Here's how the part is built. I have some questions about the finished solid (model axes, mm). A direction names the side the tool comes from. Give positions to 0.01 mm unless a question says otherwise; leave off trailing zeros. Loops run counter-clockwise (first coordinate to the right, second up) from the corner with the lowest first, then second, coordinate; pieces in that order, holes last. Notation, with made-up numbers: (37, -24.5) - (46, -24.5) arc R20 cw to (46, 7.5) - close; hole circle Ø8 at (-23, 21.5). An arc over 180 degrees is marked (long way). Use one line per item in the form item = value.
from build123d import *

# Parameters (mm, degrees)
F0_R     = 9
F0_R_2   = 3.2
F1_DEPTH = 12
F1_TAPER = 10
F3_DEPTH = 3
F4_DEPTH = 12
F5_START = 3
F5_DEPTH = 22


with BuildPart() as f1:
    # F0 (on Top) → F1 (new body)
    with BuildSketch(Plane.XY):
        Circle(F0_R)
        Polygon((-5.8312377188, 0), (-2.9156188594, 5.05), (2.9156188594, 5.05), (5.8312377188, 0), (2.9156188594, -5.05), (-2.9156188594, -5.05), align=None, mode=Mode.SUBTRACT)
        Polygon((2.9156188594, 5.05), (-2.9156188594, 5.05), (-5.8312377188, 0), (-2.9156188594, -5.05), (2.9156188594, -5.05), (5.8312377188, 0), align=None)
        Circle(F0_R_2, mode=Mode.SUBTRACT)
        Circle(F0_R_2)
    extrude(amount=F1_DEPTH, taper=F1_TAPER)

    # F2 (on Front) → F3 (join, symmetric)
    with BuildSketch(Plane.XZ):
        with BuildLine():
            Line((4.5, 12), (-4.5, 12))
            ThreePointArc((-4.5, 12), (-18.3564064606, 12), (-11.4282032303, 0))
            Line((-11.4282032303, 0), (0, 0))
            Line((0, 0), (11.4282032303, 0))
            ThreePointArc((11.4282032303, 0), (18.3564064606, 12), (4.5, 12))
        make_face()
    extrude(amount=F3_DEPTH, both=True)

    # F0 (on Top) → F4 (cut, through all)
    with BuildSketch(Plane.XY):
        Circle(F0_R_2)
    extrude(amount=F4_DEPTH, mode=Mode.SUBTRACT)

    # F0 (on Top) → F5 (cut)
    with BuildSketch(Plane.XY.offset(F5_START)):
        Polygon((2.9156188594, 5.05), (-2.9156188594, 5.05), (-5.8312377188, 0), (-2.9156188594, -5.05), (2.9156188594, -5.05), (5.8312377188, 0), align=None)
        Circle(F0_R_2, mode=Mode.SUBTRACT)
    extrude(amount=F5_DEPTH, mode=Mode.SUBTRACT)


solid = f1.part
(1) If we section it at C-C (z = 14.75): List the corners of the cut face in (x, y) for me, plus the area to 3 significant figures.
Geometry says:
outline = (-15.72, -3) - (-7.13, -3) - (-7.13, 3) - (-15.72, 3) - close; (7.13, -3) - (15.72, -3) - (15.72, 3) - (7.13, 3) - close
area = 103 mm²
(2) If I drill on probe 1 along Z at (x, y) = (3.5, 4.5); probe 2 along Z at (x, y) = (-3, 4); probe 3 along Y at (x, z) = (-11.5, 1), over which ranges is the centre line in solid material (lowest first)?
Geometry says:
probe_1 = 0 to 12
probe_2 = 0 to 3
probe_3 = -3 to 3
(3) If we section it at D-D (z = 8): List the corners of the cut face in (x, y) for me, plus the area to 3 significant figures.
Geometry says:
outline = (-19.43, -3) - (-6.97, -3) arc R7.59 ccw to (6.97, -3) - (19.43, -3) - (19.43, 3) - (6.97, 3) arc R7.59 ccw to (-6.97, 3) - (-19.43, 3) - close; hole (-5.83, 0) - (-2.92, -5.05) - (2.92, -5.05) - (5.83, 0) - (2.92, 5.05) - (-2.92, 5.05) - close
area = 237 mm²
(4) If we section it at B-B (y = -1): List the corners of the cut face in (x, z) for me.
Geometry says:
outline = (-11.43, 0) - (-3.04, 0) - (-3.04, 3) - (-5.25, 3) - (-5.25, 13.09) arc R8 ccw (long way) to start; (3.04, 0) - (11.43, 0) arc R8 ccw (long way) to (5.25, 13.09) - (5.25, 3) - (3.04, 3) - close
(5) Thinking about a two-plate mould opening in Y: for faces 3 (the flat face through (3, 2, 3)), 4 (the conical face through (-0.137, -7.926, 6.084)), 5 (the conical face through (0.137, 7.926, 6.084)), 6 (the flat face through (0, -5.05, 7)), which applies, pulls with the +Y half, pulls with the -Y half, needs draft (parallel to the pull), parting line crosses it, or undercut?
Geometry says:
face_3 = undercut
face_4 = pulls with the -Y half
face_5 = pulls with the +Y half
face_6 = undercut
(6) If we section it at A-A (x = 0): List the corners of the cut face in (y, z) for me.
Geometry says:
outline = (-9, 0) - (-3.2, 0) - (-3.2, 3) - (-5.05, 3) - (-5.05, 12) - (-6.88, 12) - close; (3.2, 0) - (9, 0) - (6.88, 12) - (5.05, 12) - (5.05, 3) - (3.2, 3) - close
(7) For P1, Ø5, axis at x = -1.5, y = -1.5, coming from the +Z side; P2, Ø1, axis at y = -5.5, z = 13, coming from the -X side; P3, Ø1.4, axis at x = -1, y = -4.5, coming from the +Z side; P4, Ø1.7, axis at x = 0.5, z = 8.5, coming from the -Y side, each with a flat end and sliding along its axis, tell me the tip position at first contact or that it passes through.
Geometry says:
P1 = 3
P2 = through
P3 = 12
P4 = -7.64
(8) For faces 1 (the flat face through (0, 5.05, 7)), 2 (the cylindrical face through (18.47, -0.04, 11.8)), which set-ups out of +Z, -Z, +X, -X, +Y, -Y let a thin tool reach every point of the face, with its end or its side?
Geometry says:
face_1 = +Z
face_2 = +Y, -Y
